Answer from the drawing. Dimensions are ordinates in mm from the lowest x, y and z of the part. A direction names the side the tool comes from. Round coordinates to 2 decimals unless told otherwise and drop trailing zeros. Loops run counter-clockwise (first coordinate to the right, second up) from the corner with the lowest first, then second, coordinate; pieces in that order, holes last.
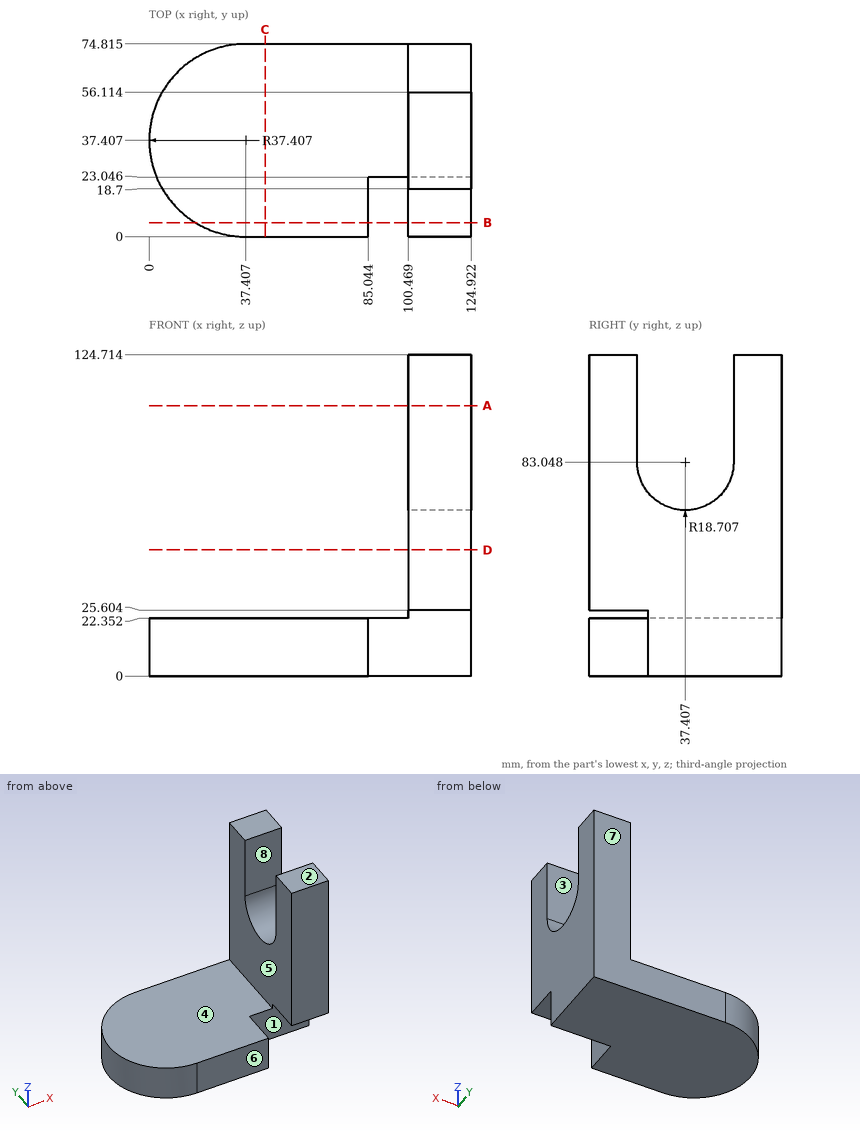
Item 1: Section D-D, the plane z = 49 is taken. Give the vertices of the cut face in (x, y) (1 decimal), plus the area to 3 significant figures.
Item 2: Each of these flat-tipped pins is pushed along its axis until it touches: P1, Ø7.5, axis at x = 112.5, z = 12.5, coming from the -Y side; P2, Ø7.5, axis at x = 116.5, z = 104.5, coming from the -Y side; P3, Ø8, axis at y = 48.5, z = 111, coming from the +X side; P4, Ø1, axis at y = 20, z = 77.5, coming from the -X side. Where does it stop, or does it pass through?
Item 3: Determine the mould class of the marked faces 5, 6, 7 and 8 for opening direction Y: pulls with the +Y half, pulls with the -Y half, needs draft (parallel to the pull), parting line crosses it, or undercut.
Item 4: For the marked faces 1, 2, 3 and 4, determine the directions among +Z, -Z, +X, -X, +Y, -Y from which every point of the face is accessible in a straight line to the end or side of a thin tool.
Item 5: Section C-C, the plane x = 45 is taken. Give the vertices of the cut face in (y, z) (1 decimal), plus the area to 3 significant figures.
Item 6: Section B-B, the plane y = 5.5 is taken. Give the vertices of the cut face in (x, z) (1 decimal).
Item 7: Straight lines are drawn through the part: line 1 (Y direction, x = 108.5, z = 110.5) (1 decimal); line 2 (X direction, y = 55, z = 40); line 3 (Z direction, x = 19, y = 58.5). For each, find the intervals that lie inside material, in ascending order.
Item 8: Section A-A, the plane z = 105 is taken. Give the vertices of the cut face in (x, y) (1 decimal).
Answer below:
1. outline: (100.5, 0) - (124.9, 0) - (124.9, 74.8) - (100.5, 74.8) - close
1. area: 1,830 mm2
2. P1: stops at y = 23.05
2. P2: stops at y = 0
2. P3: passes through
2. P4: stops at x = 100.47
3. face 5: needs draft
3. face 6: pulls with the -Y half
3. face 7: pulls with the +Y half
3. face 8: undercut
4. face 1: -Z, +X, -Y
4. face 2: +Z, +X, -X, +Y, -Y
4. face 3: +Z, +X, -X
4. face 4: +Z, -X, +Y, -Y
5. outline: (0, 0) - (74.8, 0) - (74.8, 22.4) - (0, 22.4) - close
5. area: 1,670 mm2
6. outline: (17.9, 0) - (85, 0) - (85, 22.4) - (17.9, 22.4) - close; (100.5, 25.6) - (124.9, 25.6) - (124.9, 124.7) - (100.5, 124.7) - close
7. line 1: y = 0 to 18.7, 56.1 to 74.8
7. line 2: x = 100.47 to 124.92
7. line 3: z = 0 to 22.35
8. outline: (100.5, 0) - (124.9, 0) - (124.9, 18.7) - (100.5, 18.7) - close; (100.5, 56.1) - (124.9, 56.1) - (124.9, 74.8) - (100.5, 74.8) - close
